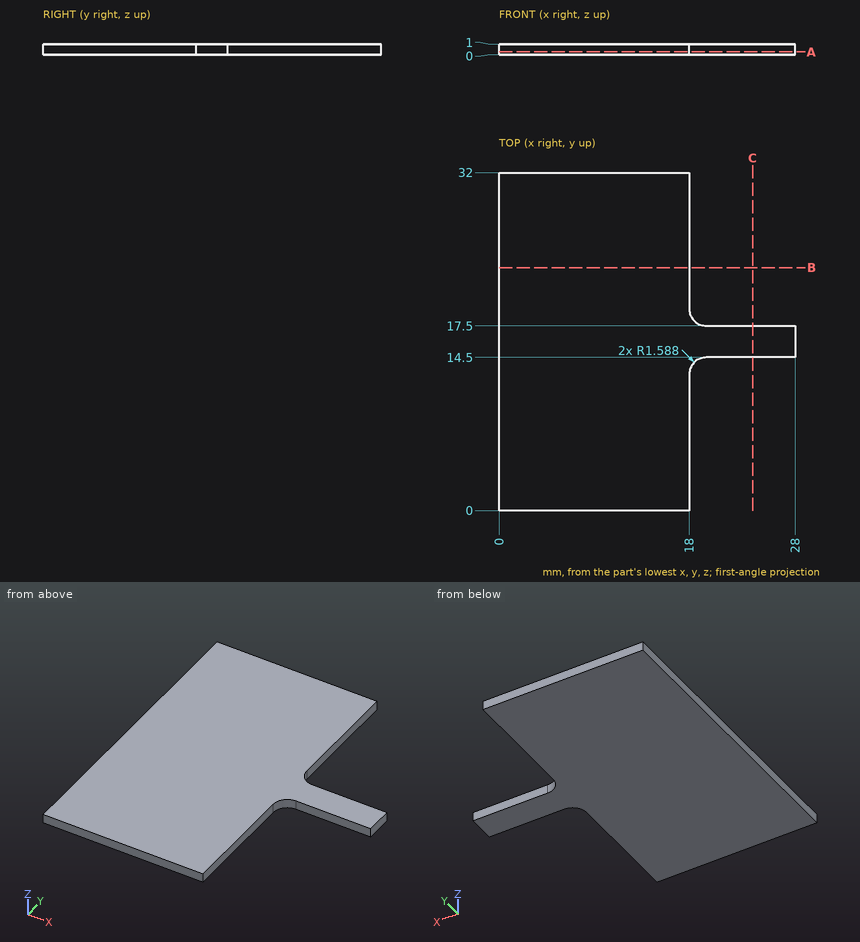
Answer from the drawing. Dimensions are ordinates in mm from the lowest x, y and z of the part. Coordinates: 2 decimals unless noted, no trailing zeros. Write each loop counter-clockwise with the first axis right and the second up, starting at its lowest first coordinate (ties: lowest second). Pieces come first, ordered by that corner, then holes. Notation, with made-up numbers: M 39.5,4 L 47.5,4 A21 ccw 47.5,36 Z; hole C 53.25,-23 d5. An arc over 180 degrees is marked long. Use one line per item in the form item = value. Start each with the question number.
1. Each of these flat-tipped pins is pushed along its axis until it touches: P1, Ø0.5, axis at y = 23.5, z = 0.5, coming from the +X side; P2, Ø1.5, axis at x = 16, y = 7.5, coming from the -Z side. Where does it stop, or does it pass through?
2. The part is cut by section A-A (z = 0.25). Give the vertices of the cut face in (x, y) (1 decimal), plus the area to 3 significant figures.
3. Straight lines are drawn through the part: probe 1 along Y at (x, z) = (26, 0.95); probe 2 along X at (y, z) = (5.5, 0.75); probe 3 along X at (y, z) = (14, 0.7). For each, find the intervals that lie inside material, in ascending order. Write a range as from..to.
4. The part is cut by section C-C (x = 24). Give the vertices of the cut face in (y, z).
5. The part is cut by section B-B (y = 23). Give the vertices of the cut face in (x, z).
Evaluation:
q1.P1 = 18
q1.P2 = 0
q2.outline = M 0,0 L 18,0 L 18,12.9 A1.6 cw 19.6,14.5 L 28,14.5 L 28,17.5 L 19.6,17.5 A1.6 cw 18,19.1 L 18,32 L 0,32 Z
q2.area = 607 mm^2
q3.probe_1 = 14.5..17.5
q3.probe_2 = 0..18
q3.probe_3 = 0..18.43
q4.outline = M 14.5,0 L 17.5,0 L 17.5,1 L 14.5,1 Z
q5.outline = M 0,0 L 18,0 L 18,1 L 0,1 Z
